Job drawing, mm, ordinate dimensions from the low corner. One solid piece. A direction names the side the tool comes from. Coordinates: 2 decimals unless noted, no trailing zeros. Loops run counter-clockwise (first coordinate to the right, second up) from the corner with the lowest first, then second, coordinate; pieces in that order, holes last. Notation, with made-up numbers: (-30, 62.5) - (-25, 62.5) arc R25 cw to (-25, 101.5) - close; hole circle Ø9 at (39.5, 48). An arc over 180 degrees is marked (long way). Use a Markdown table: item, result. Add a question column.
1) Band-saw the part on C-C (y = 23). Give the cut face in (x, z), plus the area to 3 significant figures.
2) Tool access for the marked faces 5 and 6: list every direction of +Z, -Z, +X, -X, +Y, -Y with a clear straight run to the whole face (end or side of a thin tool).
3) Pull direction X, two halves, no side cores. Call the marked faces 1, 2, 3 and 4: +X half, -X half, draft (parallel to the pull), parting line (faces both ways), or undercut.
4) Band-saw the part on B-B (x = 62). Give the cut face in (y, z), plus the area to 3 significant figures.
5) Drop flat-ended pins along their axis: P1, Ø2.5, axis at x = 147, z = 76, coming from the +Y side; P2, Ø4, axis at x = 51.5, z = 33, coming from the +Y side; P3, Ø2.5, axis at x = 120, y = 28, coming from the +Z side. Give the stop position or say it passes through.
6) Band-saw the part on A-A (z = 136.5). Give the cut face in (x, y).
7) Probe probe 1 along X at (y, z) = (28, 147.8); probe 2 along X at (y, z) = (17.5, 97). List the from-to ranges inside material, lowest first. Write a range as [from, to].
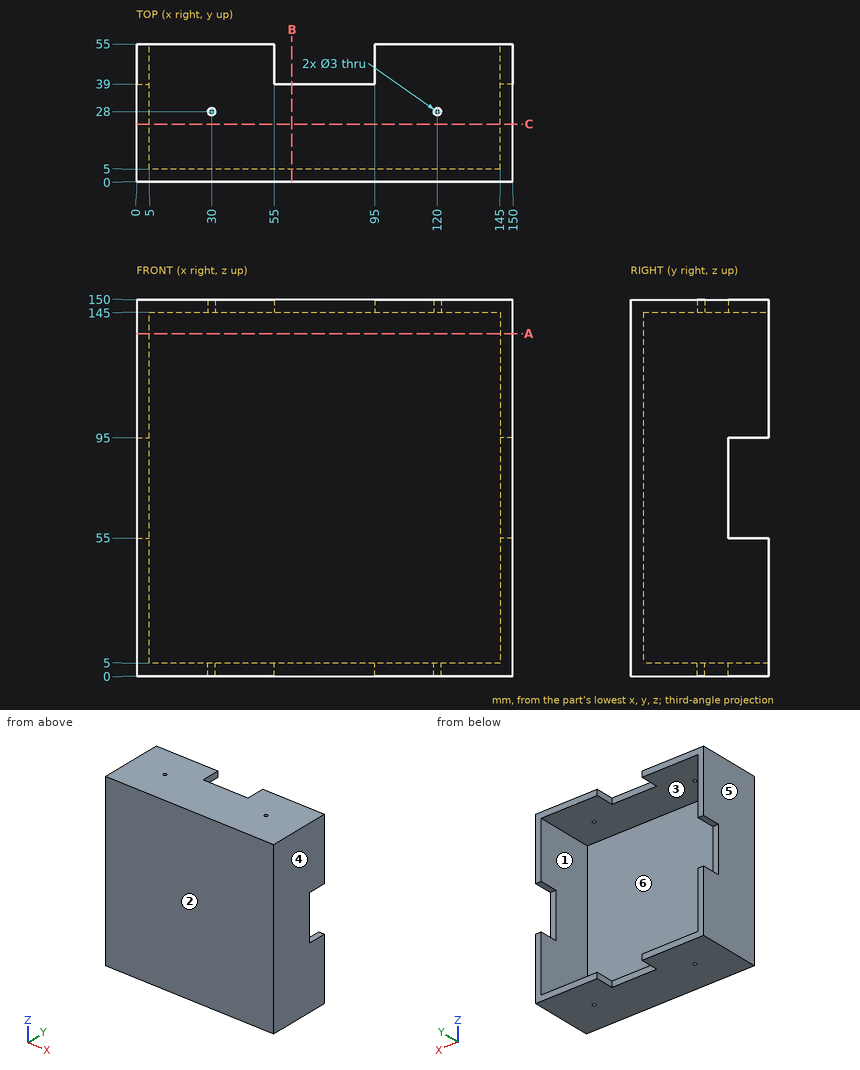
Answer block:
| question | item | result |
|---|---|---|
| 1 | outline | (0, 0) - (150, 0) - (150, 150) - (0, 150) - close; hole (5, 5) - (145, 5) - (145, 145) - (5, 145) - close |
| 1 | area | 2,900 mm2 |
| 2 | face 5 | +Z, -Z, -X, +Y, -Y |
| 2 | face 6 | +Y |
| 3 | face 1 | undercut |
| 3 | face 2 | draft |
| 3 | face 3 | undercut |
| 3 | face 4 | +X half |
| 4 | outline | (0, 0) - (39, 0) - (39, 5) - (5, 5) - (5, 145) - (39, 145) - (39, 150) - (0, 150) - close |
| 4 | area | 1,090 mm2 |
| 5 | P1 | y = 39 |
| 5 | P2 | y = 5 |
| 5 | P3 | through |
| 6 | outline | (0, 0) - (150, 0) - (150, 55) - (145, 55) - (145, 5) - (5, 5) - (5, 55) - (0, 55) - close |
| 7 | probe 1 | [0, 28.5], [31.5, 118.5], [121.5, 150] |
| 7 | probe 2 | [0, 5], [145, 150] |
